Input: dimensioned drawing with shaded views. Units: mm. Origin: part minimum x, y, z. Round coordinates to 2 decimals unless told otherwise and drop trailing zeros. Order: outer loops, then holes, each group sorted by start corner. A loop starts at its lowest first (then second) coordinate and runs counter-clockwise, first axis right, second up. Notation, with made-up numbers: (75.25, -17) -> (101.25, -17) arc R17 cw to (101.25, 1) -> close; hole circle Ø9 at (37.5, 24.25). An arc over 180 degrees is marked (long way). Use a Markdown table: item, result. Add a question column.
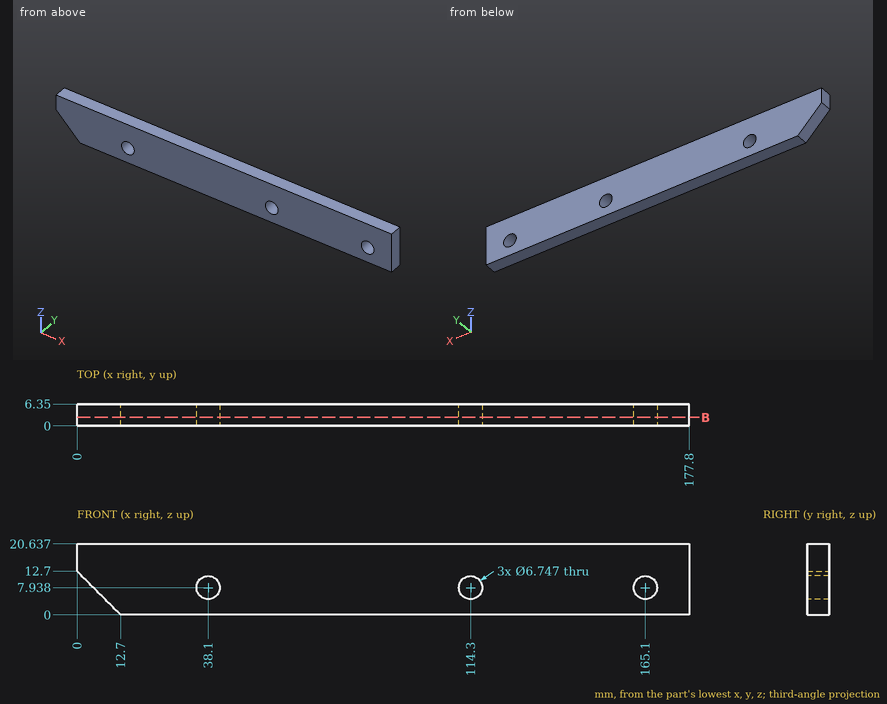
1) Section B-B on y = 2.5. Output: boundary loops of the cut face in (x, z), then the cut area to 3 significant figures.
2) Line query: probe 1 along Z at (x, y) = (114.3, 2.75) (1 decimal); probe 2 along X at (y, z) = (3, 8.5) (1 decimal); probe 3 along X at (y, z) = (4.5, 5) (1 decimal). Output: solid intervals per line, ascending. Write a range as from..to.
3) First-contact query: pin 1 Ø5.5 at (x, z) = (165.1, 7.94) entering from +Y. Flat tip, straight axial feed; report the tip coordinate or a pass-through.
Conclusion:
| question | item | result |
|---|---|---|
| 1 | outline | (0, 12.7) -> (12.7, 0) -> (177.8, 0) -> (177.8, 20.64) -> (0, 20.64) -> close; hole circle Ø6.75 at (38.1, 7.94); hole circle Ø6.75 at (114.3, 7.94); hole circle Ø6.75 at (165.1, 7.94) |
| 1 | area | 3,480 mm^2 |
| 2 | probe 1 | z = 0..4.6, 11.3..20.6 |
| 2 | probe 2 | x = 4.2..34.8, 41.4..111, 117.6..161.8, 168.4..177.8 |
| 2 | probe 3 | x = 7.7..36.4, 39.8..112.6, 116..163.4, 166.8..177.8 |
| 3 | pin 1 | passes through |
